Could you check a few things on this model? Use its own coordinates, in mm. Face numbers are marked on the shaded views. A direction names the side the tool comes from. Coordinates: 2 decimals unless noted, no trailing zeros. Loops run counter-clockwise (first coordinate to the right, second up) from the corner with the lowest first, then second, coordinate; pieces in that order, holes last. Notation, with made-up numbers: (79, 4) -> (92, 4) arc R23 ccw to (92, 34) -> close; hole circle Ø6 at (0, 59). An arc over 180 degrees is marked (long way). One line per question, with ' | ' between items.
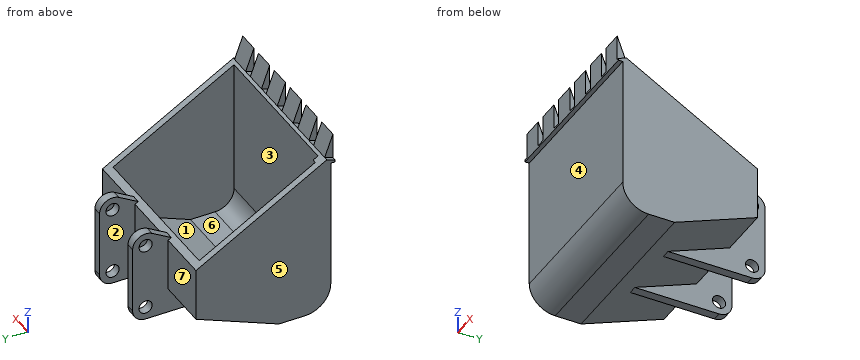
```python
from build123d import *

# Parameters (mm, degrees)
BOSS_EXTRUDE1_DEPTH = 503
SKETCH2_W           = 23
SKETCH2_H           = 139.534422093
SKETCH2_W_2         = 50
SKETCH2_W_3         = 13
CUT_EXTRUDE1_DEPTH  = 1170.669741252
SHELL1_START        = -463
SHELL1_DEPTH        = 926
SHELL1_START_2      = -440
SHELL1_2_DEPTH      = 903
BOSS_EXTRUDE2_START = 153
SKETCH4_R           = 38
BOSS_EXTRUDE2_DEPTH = 50


# Read off the part's stored shape, not the designer's step: Shell1
with BuildPart() as part:
    # Sketch1 → Boss-Extrude1 (new, symmetric)
    with BuildSketch(Plane(origin=(0, 0, 0), x_dir=(0, 0, -1), z_dir=(1, 0, 0))):
        with BuildLine():
            Line((-150, 0), (-950, 0))
            Line((-950, 0), (-499.666790032, 780))
            Line((-499.666790032, 780), (-193.666790032, 780))
            Line((-193.666790032, 780), (0, 300))
            Line((0, 300), (0, 150))
            ThreePointArc((0, 150), (-43.933982822, 43.933982822), (-150, 0))
        make_face()
        Polygon((-908, -25), (-908, 0), (-950, 0), (-936.880533213, 22.723583043), (-1068, -25), align=None)
    extrude(amount=BOSS_EXTRUDE1_DEPTH, both=True)

    # Sketch2 → Cut-Extrude1 (cut, through all)
    with BuildSketch(Plane(origin=(0, 321.173028034, 116.897422253), x_dir=(1, 0, 0), z_dir=(0, 0.9396926207859103, 0.34202014332566333))):
        with Locations((-491.5, -942.375011536)):
            Rectangle(SKETCH2_W, SKETCH2_H)
        with Locations((-335, -942.375011536)):
            Rectangle(SKETCH2_W_2, SKETCH2_H)
        with Locations((-165, -942.375011536)):
            Rectangle(SKETCH2_W_2, SKETCH2_H)
        with Locations((5, -942.375011536)):
            Rectangle(SKETCH2_W_2, SKETCH2_H)
        with Locations((175, -942.375011536)):
            Rectangle(SKETCH2_W_2, SKETCH2_H)
        with Locations((345, -942.375011536)):
            Rectangle(SKETCH2_W_2, SKETCH2_H)
        with Locations((496.5, -942.375011536)):
            Rectangle(SKETCH2_W_3, SKETCH2_H)
    extrude(amount=-CUT_EXTRUDE1_DEPTH, mode=Mode.SUBTRACT)

    # Shell1 outline → Shell1 (cut)
    with BuildSketch(Plane.YZ.offset(SHELL1_START)):
        with BuildLine():
            Line((67.944218037, 910.772387426), (40, 900.601523841))
            Line((40, 900.601523841), (40, 150))
            ThreePointArc((40, 150), (72.218254069, 72.218254069), (150, 40))
            Line((150, 40), (292.234669594, 40))
            Line((292.234669594, 40), (740, 220.660987974))
            Line((740, 220.660987974), (740, 522.7608008))
            Line((740, 522.7608008), (67.944218037, 910.772387426))
        make_face()
    extrude(amount=SHELL1_DEPTH, mode=Mode.SUBTRACT)

    # Shell1 2 outline → Shell1 2 (cut)
    with BuildSketch(Plane.YZ.offset(SHELL1_START_2)):
        Polygon((67.944218037, 910.772387426), (40, 926.905989232), (40, 900.601523841), align=None)
    extrude(amount=SHELL1_2_DEPTH, mode=Mode.SUBTRACT)

    # Sketch4 → Boss-Extrude2 (add)
    with BuildSketch(Plane(origin=(0, 0, 0), x_dir=(0, 0, -1), z_dir=(1, 0, 0)).offset(BOSS_EXTRUDE2_START)):
        with BuildLine():
            Line((-49.666790032, 423.098334058), (-49.666790032, 910))
            ThreePointArc((-49.666790032, 910), (-71.633781443, 963.033008589), (-124.666790032, 985))
            Line((-124.666790032, 985), (-509.666790032, 985))
            ThreePointArc((-509.666790032, 985), (-574.618695316, 947.5), (-574.618695316, 872.5))
            Line((-574.618695316, 872.5), (-510.440292724, 761.339745962))
            Line((-510.440292724, 761.339745962), (-499.666790032, 780))
            Line((-499.666790032, 780), (-193.666790032, 780))
            Line((-193.666790032, 780), (-49.666790032, 423.098334058))
        make_face()
        with Locations((-509.666790032, 910)):
            Circle(SKETCH4_R, mode=Mode.SUBTRACT)
        with Locations((-124.666790032, 910)):
            Circle(SKETCH4_R, mode=Mode.SUBTRACT)
    boss_extrude2 = extrude(amount=BOSS_EXTRUDE2_DEPTH)

    # Mirror1: Boss-Extrude2 across plane
    add(boss_extrude2.mirror(Plane(origin=(0, 0, 0), x_dir=(0, 0, 1), z_dir=(1, 0, 0))))


solid = part.part
```
Q1. Imagine slicing it at A-A on x = -331. Write out the boundary of the cut face in (y, z), plus the area to 3 significant figures.
Values follow:
outline: (-25, 908) -> (0, 908) -> (0, 150) arc R150 ccw to (150, 0) -> (300, 0) -> (780, 193.67) -> (780, 499.67) -> (740, 522.76) -> (740, 220.66) -> (292.23, 40) -> (150, 40) arc R110 cw to (40, 150) -> (40, 926.91) -> (22.72, 936.88) -> (-25, 919.51) -> close | area: 77,900 mm2
Q2. Imagine slicing it at B-B on y = 813.5. Write out the boundary of the cut face in (x, z).
Values follow:
outline: (-203, 49.67) -> (-153, 49.67) -> (-153, 540.56) -> (-203, 540.56) -> close; (153, 49.67) -> (203, 49.67) -> (203, 540.56) -> (153, 540.56) -> close
Q3. Imagine slicing it at D-D on y = 604. Write out the boundary of the cut face in (x, z).
Values follow:
outline: (-503, 122.66) -> (-203, 122.66) -> (-203, 49.67) -> (-153, 49.67) -> (-153, 122.66) -> (153, 122.66) -> (153, 49.67) -> (203, 49.67) -> (203, 122.66) -> (503, 122.66) -> (503, 601.28) -> (463, 601.28) -> (463, 165.79) -> (-463, 165.79) -> (-463, 601.28) -> (-503, 601.28) -> close
Q4. For pin 1 (24 mm diameter, centred on y = 0.5, z = 1027, fed in from -X); pin 2 (2 mm diameter, centred on x = -26.5, y = 414.5, fed in from +Z); pin 3 (14.5 mm diameter, centred on y = -6.5, z = 958.5, fed in from +X), each with a flat end and sliding along its axis, tell me the tip position at first contact or that it passes through.
Values follow:
pin 1: stops at x = -480 | pin 2: stops at z = 89.73 | pin 3: stops at x = 490
Q5. We'd pull the mould along Y, two halves only. Please class the marked faces 1, 2, 3 and 4: released by +Y, released by -Y, zero draft, split by the parting line, or undercut.
Values follow:
face 1: undercut | face 2: zero draft | face 3: undercut | face 4: released by -Y
Q6. For the marked faces 5, 6 and 7, which set-ups out of +Z, -Z, +X, -X, +Y, -Y let a thin tool reach every point of the face, with its end or its side?
Values follow:
face 5: +Z, -Z, -X, +Y, -Y | face 6: +Z | face 7: +Z, -Z, -X, +Y
Q7. Imagine slicing it at C-C on z = 639. Write out the boundary of the cut face in (x, y).
Values follow:
outline: (-503, 0) -> (503, 0) -> (503, 538.67) -> (463, 538.67) -> (463, 40) -> (-463, 40) -> (-463, 538.67) -> (-503, 538.67) -> close
Q8. Please list where these lines run through material, in increasing order: L1, parallel to X at y = 53.5, z = 424; L2, parallel to Y at x = 330, z = 230; L3, parallel to Y at x = -191.5, z = 514.5. Write a range as [from, to].
Values follow:
L1: x = [-503, -463], [463, 503] | L2: y = [0, 40], [740, 780] | L3: y = [0, 40], [740, 754.31], [768.37, 872.31], [947.69, 984.84]
